Input: dimensioned drawing with shaded views. Units: mm. Origin: part minimum x, y, z. A direction names the side the tool comes from. Round coordinates to 2 decimals unless told otherwise and drop trailing zeros. Loops run counter-clockwise (first coordinate to the right, second up) from the corner with the lowest first, then second, coordinate; pieces in that order, holes last.
1) Section D-D, the plane y = 6.5. Return loops of the section in (x, z).
2) First-contact query: pin 1 (1.5 mm diameter, centred on y = 3, z = 2.5, fed in from +X); pin 2 (2 mm diameter, centred on x = 43, z = 1, fed in from -Y); pin 3 (3 mm diameter, centred on x = 27.5, z = 2, fed in from +Y). Flat tips, straight axial feed; report the tip coordinate or a pass-through.
3) Section C-C, the plane x = 52.5. Return loops of the section in (y, z).
4) Access query for the marked faces 3 and 4. Directions: +Z, -Z, +X, -X, +Y, -Y. A direction counts if a zero-diameter tool reaches every point of the face in a straight line with its end or side. Return the directions, or none.
5) Section A-A, the plane y = 1. Return loops of the section in (x, z), and give its area (3 significant figures).
6) Draft query along X for the marked faces 1 and 2. Return one class per face: pulls with the +X half, pulls with the -X half, needs draft (parallel to the pull), parting line crosses it, or undercut.
7) Ray query, line 1 along X through (y, z) = (4.75, 4.95); line 2 along X through (y, z) = (6, 1.1); line 3 along Y through (x, z) = (24, 4.15). Return the intervals inside material, ascending.
8) Section B-B, the plane z = 3.9. Return loops of the section in (x, y).
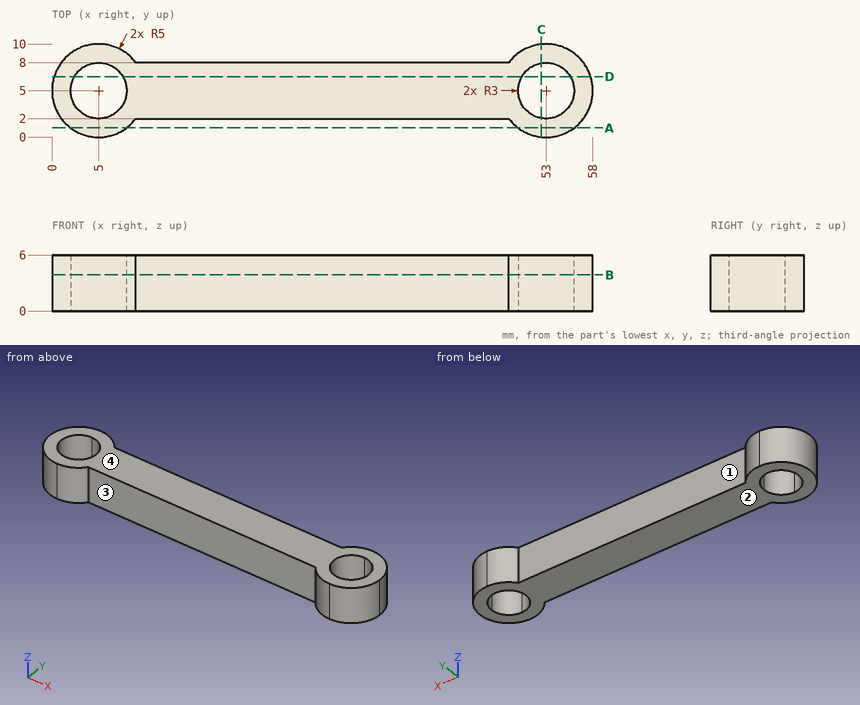
Final values:
1. outline: (0.23, 0) - (2.4, 0) - (2.4, 6) - (0.23, 6) - close; (7.6, 0) - (50.4, 0) - (50.4, 6) - (7.6, 6) - close; (55.6, 0) - (57.77, 0) - (57.77, 6) - (55.6, 6) - close
2. pin 1: stops at x = 57.84
2. pin 2: stops at y = 2
2. pin 3: stops at y = 8
3. outline: (0.03, 0) - (2.04, 0) - (2.04, 6) - (0.03, 6) - close; (7.96, 0) - (9.97, 0) - (9.97, 6) - (7.96, 6) - close
4. face 3: +Z, -Z, -Y
4. face 4: +Z, +X, -X, +Y, -Y
5. outline: (2, 0) - (8, 0) - (8, 6) - (2, 6) - close; (50, 0) - (56, 0) - (56, 6) - (50, 6) - close
5. area: 72.0 mm2
6. face 1: undercut
6. face 2: needs draft
7. line 1: x = 0.01 to 2.01, 7.99 to 50.01, 55.99 to 57.99
7. line 2: x = 0.1 to 2.17, 7.83 to 50.17, 55.83 to 57.9
7. line 3: y = 2 to 8
8. outline: (9, 2) - (49, 2) arc R5 ccw (long way) to (49, 8) - (9, 8) arc R5 ccw (long way) to start; hole circle Ø6 at (5, 5); hole circle Ø6 at (53, 5)
